CAD build for the part. Positions are in the model's coordinates, mm. Face numbers are marked on the shaded views. A direction names the side the tool comes from. Coordinates: 2 decimals unless noted, no trailing zeros. Order: outer loops, then holes, each group sorted by start corner. A loop starts at its lowest first (then second) coordinate and runs counter-clockwise, first axis right, second up. Notation, with made-up numbers: (56, 44) - (108, 44) arc R21 ccw to (108, 76) - close; hole circle Ø3 at (-22, 70). An arc over 180 degrees is marked (long way). Return JSON: item names as keys, results as strings.
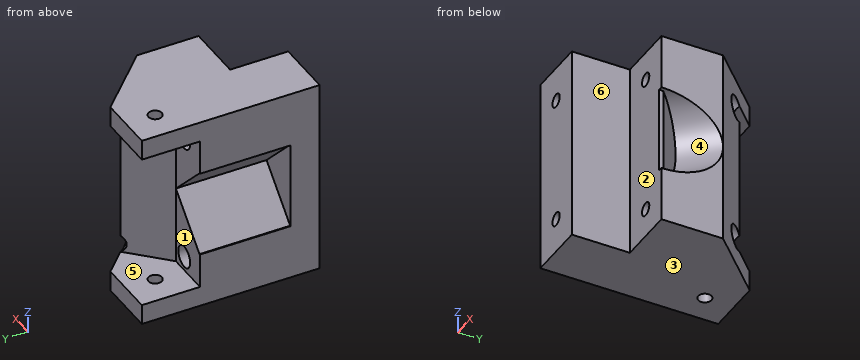
from build123d import *

# Parameters (mm, degrees)
AUFSATZ_LINEAR_AUSTRAGEN1_DEPTH = 68
SKIZZE4_R                       = 15
SCHNITT_LINEAR_AUSTRAGEN1_DEPTH = 20
SKIZZE9_W                       = 27.635547715
SKIZZE9_H                       = 54
SCHNITT_LINEAR_AUSTRAGEN6_DEPTH = 20
SKIZZE5_R                       = 2.3
SCHNITT_LINEAR_AUSTRAGEN2_DEPTH = 20
SKIZZE6_R                       = 3.75
SCHNITT_LINEAR_AUSTRAGEN3_DEPTH = 96.723933406
SKIZZE7_R                       = 2.3
SCHNITT_LINEAR_AUSTRAGEN4_DEPTH = 20
SKIZZE8_R                       = 3.75
SCHNITT_LINEAR_AUSTRAGEN5_DEPTH = 86.991530335
FASE1_SIZE                      = 12.36
SKIZZE10_W                      = 15.275547715
SKIZZE10_H                      = 30
SCHNITT_LINEAR_AUSTRAGEN7_DEPTH = 31.213203436
FASE2_SIZE                      = 15
SKIZZE12_R                      = 2.3
SCHNITT_LINEAR_AUSTRAGEN8_DEPTH = 100.855176505
FASE3_SIZE                      = 2
FASE3_SIZE2                     = 1.414213562


with BuildPart() as part:
    # Skizze1 → Aufsatz-Linear austragen1 (new body)
    with BuildSketch(Plane.XY):
        Polygon((0, 0), (20, 0), (20, 20), (40, 20), (40, 41.213203436), (20, 61.213203436), (0, 61.213203436), align=None)
    extrude(amount=-AUFSATZ_LINEAR_AUSTRAGEN1_DEPTH)

    # Skizze4 → Schnitt-Linear austragen1 (cut)
    with BuildSketch(Plane(origin=(30, 30, 0), x_dir=(0, 0, 1), z_dir=(-0.7071067811865507, -0.7071067811865445, -1.0200465955922179e-15))):
        with Locations((-34, -14.142135624)):
            Circle(SKIZZE4_R)
    extrude(amount=-SCHNITT_LINEAR_AUSTRAGEN1_DEPTH, mode=Mode.SUBTRACT)

    # Skizze9 → Schnitt-Linear austragen6 (cut)
    with BuildSketch(Plane(origin=(0, 61.213203436, 0), x_dir=(1, 0, 0), z_dir=(0, 1, 0))):
        with Locations((13.817773858, 34)):
            Rectangle(SKIZZE9_W, SKIZZE9_H)
    extrude(amount=-SCHNITT_LINEAR_AUSTRAGEN6_DEPTH, mode=Mode.SUBTRACT)

    # Skizze5 → Schnitt-Linear austragen2 (cut)
    with BuildSketch(Plane(origin=(0, 7, 0), x_dir=(-1, 0, 0), z_dir=(0, -1, 0))):
        with Locations(Location((-10, 56, 0), (0, 0, 180))):
            Circle(SKIZZE5_R)
        with Locations((-10, 12)):
            Circle(SKIZZE5_R)
    extrude(amount=SCHNITT_LINEAR_AUSTRAGEN2_DEPTH, mode=Mode.SUBTRACT)

    # Skizze6 → Schnitt-Linear austragen3 (cut, through all)
    with BuildSketch(Plane(origin=(0, 7, 0), x_dir=(-1, 0, 0), z_dir=(0, -1, 0))):
        with Locations(Location((-10, 56, 0), (0, 0, 180))):
            Circle(SKIZZE6_R)
        with Locations(Location((-10, 12, 0), (0, 0, 180))):
            Circle(SKIZZE6_R)
    extrude(amount=-SCHNITT_LINEAR_AUSTRAGEN3_DEPTH, mode=Mode.SUBTRACT)

    # Skizze7 → Schnitt-Linear austragen4 (cut)
    with BuildSketch(Plane(origin=(0, 27, 0), x_dir=(-1, 0, 0), z_dir=(0, -1, 0))):
        with Locations(Location((-30, 58, 0), (0, 0, 180))):
            Circle(SKIZZE7_R)
        with Locations((-30, 10)):
            Circle(SKIZZE7_R)
    extrude(amount=SCHNITT_LINEAR_AUSTRAGEN4_DEPTH, mode=Mode.SUBTRACT)

    # Skizze8 → Schnitt-Linear austragen5 (cut, through all)
    with BuildSketch(Plane(origin=(0, 27, 0), x_dir=(-1, 0, 0), z_dir=(0, -1, 0))):
        with Locations(Location((-30, 58, 0), (0, 0, 180))):
            Circle(SKIZZE8_R)
        with Locations(Location((-30, 10, 0), (0, 0, 180))):
            Circle(SKIZZE8_R)
    extrude(amount=-SCHNITT_LINEAR_AUSTRAGEN5_DEPTH, mode=Mode.SUBTRACT)

    # Fase1
    fase1_edges = [part.edges().sort_by_distance(p)[0] for p in [
        (27.635547715, 41.213203436, -34),
    ]]
    chamfer(fase1_edges, length=FASE1_SIZE)

    # Skizze10 → Schnitt-Linear austragen7 (cut)
    with BuildSketch(Plane(origin=(0, 41.213203436, 0), x_dir=(1, 0, 0), z_dir=(0, 1, 0))):
        with Locations((7.637773858, 34)):
            Rectangle(SKIZZE10_W, SKIZZE10_H)
    extrude(amount=-SCHNITT_LINEAR_AUSTRAGEN7_DEPTH, mode=Mode.SUBTRACT)

    # Fase2
    fase2_edges = [part.edges().sort_by_distance(p)[0] for p in [
        (15.275547715, 25.606601718, -19),
        (15.275547715, 25.606601718, -49),
    ]]
    chamfer(fase2_edges, length=FASE2_SIZE - 0.0001)  # a hair under: the kernel refuses the full size

    # Skizze12 → Schnitt-Linear austragen8 (cut, through all)
    with BuildSketch(Plane(origin=(0, 0, -68), x_dir=(-1, 0, 0), z_dir=(0, 0, -1))):
        with Locations((-10, 51.213203436)):
            Circle(SKIZZE12_R)
    extrude(amount=-SCHNITT_LINEAR_AUSTRAGEN8_DEPTH, mode=Mode.SUBTRACT)

    # Fase3
    fase3_edges = [part.edges().sort_by_distance(p)[0] for p in [
        (40, 20, -34),
    ]]
    fase3_side = [part.faces().sort_by_distance(p)[0] for p in [
        (35.498418419, 24.501581581, -34),
    ]]
    chamfer(fase3_edges, length=FASE3_SIZE, length2=FASE3_SIZE2, reference=fase3_side[0])


solid = part.part
Item 1: Band-saw the part on D-D, the plane x = 22. List the corners of the cut face in (y, z), then the cut area to 3 significant figures.
Findings below:
{"outline": "(20, -68) - (59.21, -68) - (59.21, -61) - (47.94, -61) - (47.94, -7) - (59.21, -7) - (59.21, 0) - (20, 0) - close", "area": "2,060 mm²"}
Item 2: Band-saw the part on B-B, the plane z = -4.5. List the corners of the cut face in (x, y).
Findings below:
{"outline": "(0, 0) - (20, 0) - (20, 20) - (40, 20) - (40, 41.21) - (20, 61.21) - (0, 61.21) - close; hole circle Ø4.6 at (10, 51.21)"}
Item 3: Mould opens along Z. For the marked faces 1, 2 and 3 say: released by +Z, released by -Z, zero draft, split by the parting line, or undercut.
Findings below:
{"face 1": "undercut", "face 2": "zero draft", "face 3": "released by -Z"}
Item 4: Band-saw the part on A-A, the plane y = 11.5. Count the separate pieces of the cut face and the enclosed holes in it, then the cut area to 3 significant figures.
Findings below:
{"separate pieces": "1", "enclosed holes": "2", "area": "1,040 mm²"}
Item 5: Which spindle directions (+Z, -Z, +X, -X, +Y, -Y) get a long thin tool onto all of the face, cutting with end or side? Do the marked faces 4, 5 and 6. Say none if no direction does.
Findings below:
{"face 4": "+X", "face 5": "-X, +Y", "face 6": "+Z, -Z, +X, -Y"}
Item 6: Drop flat-ended pins along their axis: P1, Ø4, axis at x = 10.5, z = -10.5, coming from the +Y side; P2, Ø1, axis at y = 31.5, z = -46, coming from the -X side; P3, Ø12, axis at x = 6, z = -45, coming from the +Y side; P4, Ø16, axis at x = 27.5, z = -18.5, coming from the -Y side. Give the stop position or say it passes through.
Findings below:
{"P1": "stops at y = 7", "P2": "stops at x = 2.78", "P3": "stops at y = 41.21", "P4": "stops at y = 0"}
Item 7: Wall check: L1, parallel to Z at x = 30, y = 21.75; L2, parallel to Z at x = 30, y = 44.5; L3, parallel to Y at x = 10, z = -3.25. Give the ranges that are in metal, low to high. Write a range as [from, to].
Findings below:
{"L1": "z = [-68, -60.3], [-55.7, -12.3], [-7.7, 0]", "L2": "z = [-68, -61.75], [-54.25, -13.75], [-6.25, 0]", "L3": "y = [0, 48.91], [53.51, 61.21]"}
